Verification items for the finished model (mm, model axes). A direction names the side the tool comes from. Give positions to 0.01 mm unless a question says otherwise; leave off trailing zeros. Order: outer loops, then holes, each group sorted by start corner. A loop starts at its lowest first (then second) coordinate and runs counter-clockwise, first axis right, second up. Notation, with made-up numbers: M 89,51.5 L 116,51.5 A19 cw 116,64.5 Z; hole C 59,6.5 d5. An arc over 180 degrees is marked long. Answer as a JSON object with one key per item and string values.
```python
from build123d import *

# Parameters (mm, degrees)
PAD_DEPTH   = 7
THICKNESS_T = -2


with BuildPart() as part:
    # Sketch → Pad (new body)
    with BuildSketch(Plane.XY):
        Polygon((0, 0), (40, 0), (40, 16.2), (16.2, 16.2), (16.2, 40), (0, 40), align=None)
    extrude(amount=PAD_DEPTH)

    # Thickness
    thickness_openings = [part.faces().sort_by_distance(p)[0] for p in [
        (15.560815, 15.560815, 7),
        (40, 8.1, 3.5),
        (8.1, 40, 3.5),
    ]]
    offset(amount=THICKNESS_T, openings=thickness_openings)


solid = part.part
```
Q1. Gauge pin test, flat ends, axial feed: pin 1 Ø2.5 at (x, z) = (26.5, 4) entering from +Y; pin 2 Ø3.5 at (y, z) = (33, 3) entering from +X. Record the tip position at first contact, or that the pin passes through.
Resolved:
{"pin 1": "stops at y = 16.2", "pin 2": "stops at x = 16.2"}
Q2. Section check B-B on y = 35. Record the cut outline in (x, z), then the cut area to 3 significant figures.
Resolved:
{"outline": "M 0,0 L 16.2,0 L 16.2,7 L 14.2,7 L 14.2,2 L 2,2 L 2,7 L 0,7 Z", "area": "52.4 mm²"}
Q3. Tool access check on faces 1 (the face through (12, 17, 2)), 2 (the face through (2, 21, 4)), 3 (the face through (16.2, 28, 3)), 4 (the face through (21, 2, 4)). Record the directions out of +Z, -Z, +X, -X, +Y, -Y that give a thin tool (end or side, any length) a straight path to the whole face; none if there is none.
Resolved:
{"face 1": "+Z", "face 2": "+Z, +Y", "face 3": "+Z, -Z, +X, +Y", "face 4": "+Z, +X"}
Q4. Material ranges on L1, parallel to X at y = 37.5, z = 3; L2, parallel to Z at x = 22, y = 13.5, recorded low to high.
Resolved:
{"L1": "x = 0 to 2, 14.2 to 16.2", "L2": "z = 0 to 2"}
Q5. Section check D-D on y = 5.5. Record the cut outline in (x, z), then the cut area to 3 significant figures.
Resolved:
{"outline": "M 0,0 L 40,0 L 40,2 L 2,2 L 2,7 L 0,7 Z", "area": "90.0 mm²"}
Q6. Release check for a two-part mould opening along Y. For faces 5 (the face through (28, 14.2, 4)), 6 (the face through (15, 16, 0)), 7 (the face through (8, 40, 1)), 8 (the face through (14.8, 14.77, 4.54)) record: +Y half, -Y half, draft (parallel to the pull), parting line (faces both ways), or undercut.
Resolved:
{"face 5": "undercut", "face 6": "draft", "face 7": "+Y half", "face 8": "undercut"}
Q7. Section check A-A on z = 3.5. Record the cut outline in (x, y).
Resolved:
{"outline": "M 0,0 L 40,0 L 40,2 L 2,2 L 2,40 L 0,40 Z; M 14.2,16.2 A2 ccw 16.2,14.2 L 40,14.2 L 40,16.2 L 16.2,16.2 L 16.2,40 L 14.2,40 Z"}
